from build123d import *

# Parameters (mm, degrees)
F1_DEPTH  = 16
F2_W      = 70
F2_H      = 3
F3_DEPTH  = 2
F4_W      = 50
F4_H      = 12
F5_DEPTH  = 2
F6_R      = 1
F9_DEPTH  = 2
F11_DEPTH = 38.001
F13_D     = 4
F14_R     = 3
F14_R_2   = 2
F15_DEPTH = 5
F16_R     = 3


# Not quite as in the source:
# - a pattern or mirror of a feature is missing from the dataset's text; its kind, count and spacing are read off the source's solid


with BuildPart() as f1:
    # F0 (on Front) → F1 (new body)
    with BuildSketch(Plane.XZ):
        with BuildLine():
            Line((94, 11), (0, 11))
            ThreePointArc((0, 11), (-11, 0), (0, -11))
            Line((0, -11), (19, -11))
            ThreePointArc((19, -11), (21.7648271935, -11.8339790459), (23.607331209, -14.0577077639))
            ThreePointArc((23.607331209, -14.0577077639), (48.6917034204, -45.0930519948), (86.4506679072, -58.0034711071))
            ThreePointArc((86.4506679072, -58.0034711071), (93.1291053538, -58.9355091014), (98.8304523125, -62.5361846502))
            Line((98.8304523125, -62.5361846502), (100.1194642859, -61))
            ThreePointArc((100.1194642859, -61), (93.803453137, -57.0525770858), (86.4301074938, -56))
            ThreePointArc((86.4301074938, -56), (49.7895156694, -43.4202136678), (25.4502636926, -13.2807908695))
            ThreePointArc((25.4502636926, -13.2807908695), (22.8707580709, -10.1675706642), (19, -9))
            Line((19, -9), (0, -9))
            ThreePointArc((0, -9), (-9, 0), (0, 9))
            Line((0, 9), (94, 9))
            Line((94, 9), (94, 11))
        make_face()
    extrude(amount=F1_DEPTH)

    # F2 (on face) → F3 (join)
    with BuildSketch(Plane.XY.offset(11)):
        with Locations((59, -17.5)):
            Rectangle(F2_W, F2_H)
    extrude(amount=-F3_DEPTH)

    # F4 (on face) → F5 (join)
    with BuildSketch(Plane.XZ.offset(19)):
        with Locations((69, 3)):
            Rectangle(F4_W, F4_H)
    extrude(amount=-F5_DEPTH)

    # F6
    f6_edges = [f1.edges().sort_by_distance(p)[0] for p in [
        (59, -19, 11),
        (69, -17, 9),
    ]]
    fillet(f6_edges, radius=F6_R)

    # F7: F1 across plane


with BuildPart() as f1_1:
    add(f1.part)
    add(f1.part.mirror(Plane.XZ))

    # F8 (on face) → F9 (cut)
    with BuildSketch(Plane.XY.offset(11)):
        with BuildLine():
            Line((94, 12), (34, 12))
            ThreePointArc((34, 12), (22, 0), (34, -12))
            Line((34, -12), (94, -12))
            Line((94, -12), (94, 12))
        make_face()
    extrude(amount=-F9_DEPTH, mode=Mode.SUBTRACT)

    # F10 (on face) → F11 (cut, through all)
    with BuildSketch(Plane.XZ.offset(19)):
        with BuildLine():
            ThreePointArc((50, 5), (47, 2), (50, -1))
            Line((50, -1), (70, -1))
            ThreePointArc((70, -1), (73, 2), (70, 5))
            Line((70, 5), (50, 5))
        make_face()
    extrude(amount=-F11_DEPTH, mode=Mode.SUBTRACT)

    # F13 (through all)
    with Locations(Plane.XZ.offset(19)):
        with Locations((80, 3)):
            Hole(F13_D / 2)

    # F14 (on face) → F15 (join)
    with BuildSketch(Plane(origin=(0, -17, 0), x_dir=(-1, 0, 0), z_dir=(0, 1, 0))):
        with Locations((-80, 3)):
            Circle(F14_R)
        with Locations((-80, 3)):
            Circle(F14_R_2, mode=Mode.SUBTRACT)
    f15 = extrude(amount=F15_DEPTH)

    # F15_copies: F15 across plane
    add(f15.mirror(Plane.ZX))

    # F16
    f16_edges = [f1_1.edges().sort_by_distance(p)[0] for p in [
        (94, 18, -3),
        (44, 18, -3),
        (44, -18, -3),
        (94, -18, -3),
    ]]
    fillet(f16_edges, radius=F16_R)


solid = f1_1.part
Can you work these out from the model? Positions are in its coordinate system, mm. A direction names the side the tool comes from. Coordinates: 2 decimals unless noted, no trailing zeros. Write each loop counter-clockwise with the first axis right and the second up, starting at its lowest first coordinate (ties: lowest second). Pieces come first, ordered by that corner, then holes.
Q1. For P1, Ø4, axis at x = 19, y = 9, coming from the -Z side; P2, Ø0.6, axis at x = 60, y = 18, coming from the -Z side; P3, Ø8, axis at y = 15, z = -38.5, coming from the -X side; P4, Ø8, axis at y = 10.5, z = -1.5, coming from the -X side, each with a flat end and sliding along its axis, tell me the tip position at first contact or that it passes through.
Results found:
P1: stops at z = -11.42
P2: stops at z = -3
P3: stops at x = 36.66
P4: stops at x = -11
Q2. Imagine slicing it at B-B, the plane x = 60. List the corners of the cut face in (y, z) for me.
Results found:
outline: (-19, -3) - (-17, -3) - (-17, -1) - (-19, -1) - close; (-19, 5) - (-17, 5) - (-17, 8) arc R1 cw to (-16, 9) - (-12, 9) - (-12, 11) - (-18, 11) arc R1 ccw to (-19, 10) - close; (-16, -51.56) - (16, -51.56) - (16, -49.36) - (-16, -49.36) - close; (12, 9) - (16, 9) arc R1 cw to (17, 8) - (17, 5) - (19, 5) - (19, 10) arc R1 ccw to (18, 11) - (12, 11) - close; (17, -3) - (19, -3) - (19, -1) - (17, -1) - close
Q3. Imagine slicing it at D-D, the plane x = 88.5. List the corners of the cut face in (y, z) for me, plus the area to 3 significant figures.
Results found:
outline: (-19, -3) - (-17, -3) - (-17, 8) arc R1 cw to (-16, 9) - (-12, 9) - (-12, 11) - (-18, 11) arc R1 ccw to (-19, 10) - close; (-16, -57.98) - (16, -57.98) - (16, -55.98) - (-16, -55.98) - close; (12, 9) - (16, 9) arc R1 cw to (17, 8) - (17, -3) - (19, -3) - (19, 10) arc R1 ccw to (18, 11) - (12, 11) - close
area: 140 mm2
Q4. Imagine slicing it at C-C, the plane y = 0. List the corners of the cut face in (x, z) for me.
Results found:
outline: (0, -11) - (19, -11) arc R5 cw to (23.61, -14.06) arc R72 ccw to (86.45, -58) arc R16 cw to (98.83, -62.54) - (100.12, -61) arc R18 ccw to (86.43, -56) arc R70 cw to (25.45, -13.28) arc R7 ccw to (19, -9) - (0, -9) arc R9 cw to (0, 9) - (22, 9) - (22, 11) - (0, 11) arc R11 ccw to start
Q5. Imagine slicing it at A-A, the plane y = 14. List the corners of the cut face in (x, z) for me.
Results found:
outline: (0, -11) - (19, -11) arc R5 cw to (23.61, -14.06) arc R72 ccw to (86.45, -58) arc R16 cw to (98.83, -62.54) - (100.12, -61) arc R18 ccw to (86.43, -56) arc R70 cw to (25.45, -13.28) arc R7 ccw to (19, -9) - (0, -9) arc R9 cw to (0, 9) - (94, 9) - (94, 11) - (0, 11) arc R11 ccw to start; circle Ø6 at (80, 3); hole circle Ø4 at (80, 3)
Q6. Please list where these lines run through material, in increasing order: L1, parallel to Z at x = 80, y = -15; L2, parallel to Z at x = 80, y = 17.25; L3, parallel to Z at x = 86, y = -14.5.
Results found:
L1: z = -57.4 to -55.38, 0 to 1, 5 to 6, 9 to 11
L2: z = -3 to 1, 5 to 11
L3: z = -57.98 to -55.98, 9 to 11
Q7. If we mould it in two halves opening along Y, with no side actions, what happens to faces 5 (the face through (83, 15, 3)), 6 (the face through (10, 0, -9)), 7 (the face through (28, -16, -20))? For each: +Y half, -Y half, draft (parallel to the pull), parting line (faces both ways), or undercut.
Results found:
face 5: undercut
face 6: draft
face 7: -Y half
Q8. Which directions (+Z, -Z, +X, -X, +Y, -Y) give clear straight access to the entire face, cutting with the end or side of a thin tool? Please do faces 1 (the face through (94, 18, 7)), 2 (the face through (79, -12, 1)), 3 (the face through (25, -9, 9)), 4 (the face through (73, -18, 2)).
Results found:
face 1: +Z, +X, +Y, -Y
face 2: +Z, +X
face 3: none
face 4: +Y, -Y
